```python
from build123d import *

# Parameters (mm, degrees)
F0_R     = 11.519276
F0_R_2   = 9.9
F1_DEPTH = 7
F2_SIZE  = 0.508
F3_SIZE  = 0.508


with BuildPart() as f1:
    # F0 (on Top) → F1 (new body)
    with BuildSketch(Plane.XY):
        Circle(F0_R)
        Circle(F0_R_2, mode=Mode.SUBTRACT)
    extrude(amount=F1_DEPTH)

    # F2
    f2_edges = [f1.edges().sort_by_distance(p)[0] for p in [
        (-9.9, 0, 0),
        (-9.9, 0, 7),
    ]]
    chamfer(f2_edges, length=F2_SIZE)

    # F3
    f3_edges = [f1.edges().sort_by_distance(p)[0] for p in [
        (-11.519276, 0, 7),
        (-11.519276, 0, 0),
    ]]
    chamfer(f3_edges, length=F3_SIZE)


solid = f1.part
```
Source: CAD feature listing. Evaluate the final solid. Frame: model axes, mm. Coordinates: 2 decimals unless noted, no trailing zeros. Order: outer loops, then holes, each group sorted by start corner. A loop starts at its lowest first (then second) coordinate and runs counter-clockwise, first axis right, second up. Notation, with made-up numbers: M -21.75,89.25 L 0.25,89.25 A21 ccw 0.25,118.25 Z; hole C 46.5,24.25 d5. An arc over 180 degrees is marked long. Write each question's results on one line, items separated by ' | '. Start each with the question number.
1) Section query C-C (z = 1.75). Return the cut outline in (x, y).
2) Draft query along X for faces 1 (the face through (-2.497, -11.245, 3.458)), 2 (the face through (9.443, 2.974, 3.458)), 3 (the face through (8, 7, 0)). Return one class per face: released by +X, released by -X, zero draft, split by the parting line, or undercut.
3) Contact query for flat-ended pins moving along their axis: pin 1 Ø10 at (x, y) = (-1.5, 3) entering from -Z; pin 2 Ø2 at (y, z) = (5, 4) entering from +X; pin 3 Ø1 at (y, z) = (-7, 3.5) entering from -X; pin 4 Ø4 at (x, z) = (0.5, 2.5) entering from -Y. Output: stop coordinate, or through.
4) Line query: line 1 (Y direction, x = 0, z = 3); line 2 (Y direction, x = 8, z = 5.75); line 3 (X direction, y = -8.25, z = 6.75). Output: solid intervals per line, ascending. Write a range as from..to.
5) Section query A-A (y = 0). Return the cut outline in (x, z), plus the area to 3 significant figures.
Answers:
1) outline: C 0,0 d23.04; hole C 0,0 d19.8
2) face 1: split by the parting line | face 2: undercut | face 3: zero draft
3) pin 1: passes through | pin 2: stops at x = 10.8 | pin 3: stops at x = -9.51 | pin 4: stops at y = -11.52
4) line 1: y = -11.52..-9.9, 9.9..11.52 | line 2: y = -8.29..-5.83, 5.83..8.29 | line 3: x = -7.67..-5.93, 5.93..7.67
5) outline: M -11.52,0.51 L -11.01,0 L -10.41,0 L -9.9,0.51 L -9.9,6.49 L -10.41,7 L -11.01,7 L -11.52,6.49 Z; M 9.9,0.51 L 10.41,0 L 11.01,0 L 11.52,0.51 L 11.52,6.49 L 11.01,7 L 10.41,7 L 9.9,6.49 Z | area: 21.6 mm^2
